Input: part model. Units: mm. Frame: model coordinates. A direction names the side the tool comes from. Give positions to 0.01 mm unless a question says otherwise; leave off trailing zeros. Loops run counter-clockwise (first coordinate to the right, second up) from the corner with the lowest first, then second, coordinate; pieces in that order, holes last.
from build123d import *

# Parameters (mm, degrees)
F1_DEPTH = 69.85
F3_D     = 3.302
F5_D     = 3.302


with BuildPart() as f1:
    # F0 (on Right) → F1 (new body)
    with BuildSketch(Plane.YZ):
        Polygon((0, 12.7), (0, 0), (44.45, 0), (44.45, 3.175), (3.175, 3.175), (3.175, 12.7), align=None)
    extrude(amount=F1_DEPTH)

    # F3 (through all)
    with Locations(Plane(origin=(0, 0, 0), x_dir=(1, 0, 0), z_dir=(0, 0, -1))):
        with Locations((6.35, -14.351), (63.5, -14.351)):
            Hole(F3_D / 2)

    # F5 (through all)
    with Locations(Plane.XZ):
        with Locations((17.018, 6.35)):
            Hole(F5_D / 2)


solid = f1.part
(1) Cut plane A-A (x = 6.35). Return the cut outline in (y, z) (3 decimals), and give its area (3 significant figures).
Values follow:
outline: (0, 0) - (12.7, 0) - (12.7, 3.175) - (3.175, 3.175) - (3.175, 12.7) - (0, 12.7) - close; (16.002, 0) - (44.45, 0) - (44.45, 3.175) - (16.002, 3.175) - close
area: 161 mm2
(2) Cut plane D-D (x = 60). Return the cut outline in (y, z) (3 decimals), and give its area (3 significant figures).
Values follow:
outline: (0, 0) - (44.45, 0) - (44.45, 3.175) - (3.175, 3.175) - (3.175, 12.7) - (0, 12.7) - close
area: 171 mm2
(3) Reachability of faces 4 (the flat face through (34, 3.175, 8)), 5 (the flat face through (34, 44.45, 2)) from +Z, -Z, +X, -X, +Y, -Y: full face, straight path, thin tool, end or side. Return the list, or none.
Values follow:
face 4: +Z, +X, -X, +Y
face 5: +Z, -Z, +X, -X, +Y
(4) Mould query, pull axis X, two halves, no side actions, for faces 1 (the flat face through (34, 22, 0)), 2 (the flat face through (0, 19, 3)), 3 (the cylindrical face through (65.15, 14.28, 1.61)). Classes: +X half, -X half, draft (parallel to the pull), parting line (faces both ways), or undercut.
Values follow:
face 1: draft
face 2: -X half
face 3: undercut
(5) Cut plane B-B (z = 6.35). Return the cut outline in (x, y) (3 decimals), and give its area (3 significant figures).
Values follow:
outline: (0, 0) - (15.367, 0) - (15.367, 3.175) - (0, 3.175) - close; (18.669, 0) - (69.85, 0) - (69.85, 3.175) - (18.669, 3.175) - close
area: 211 mm2
(6) Pin query (flat end, axial travel): pin 1 Ø4 at (x, z) = (36, 8.5) entering from -Y; pin 2 Ø12 at (x, y) = (38, 9.5) entering from +Z (3 decimals); pin 3 Ø4.5 at (x, z) = (17.018, 6.35) entering from +Y (3 decimals); pin 4 Ø3 at (x, y) = (63.5, 14.351) entering from -Z. Return the tip coordinate at first contact, or that it passes through.
Values follow:
pin 1: stops at y = 0
pin 2: stops at z = 3.175
pin 3: stops at y = 3.175
pin 4: passes through
(7) Cut plane C-C (z = 10.25). Return the cut outline in (x, y) (3 decimals).
Values follow:
outline: (0, 0) - (69.85, 0) - (69.85, 3.175) - (0, 3.175) - close
(8) Ray query, probe 1 along Y at (x, z) = (63.5, 2.4); probe 2 along Z at (x, y) = (51, 18) (3 decimals). Return the intervals inside material, ascending.
Values follow:
probe 1: y = 0 to 12.7, 16 to 44.45
probe 2: z = 0 to 3.175
